```python
from build123d import *

# Parameters (mm, degrees)
F1_DEPTH  = 50.8
F2_R      = 31.75
F3_DEPTH  = 19.05
F4_R      = 12.7
F5_DEPTH  = 38.1
F6_R      = 22.225
F7_DEPTH  = 25.4
F11_R     = 10.16
F12_DEPTH = 25.4


# Not quite as in the source:
# - a fillet or chamfer that OpenCascade refuses, or shapes differently, is made with other operations: its cross-section is extruded or revolved along the edge and cut away or added


with BuildPart() as f1:
    # F0 (on Top) → F1 (new body)
    with BuildSketch(Plane.XY):
        Polygon((76.6512806053, -31.75), (76.6512806053, 31.75), (31.75, 76.6512806053), (-31.75, 76.6512806053), (-76.6512806053, 31.75), (-76.6512806053, -31.75), (-31.75, -76.6512806053), (31.75, -76.6512806053), align=None)
    extrude(amount=F1_DEPTH)

    # F2 (on face) → F3 (cut)
    with BuildSketch(Plane.XY.offset(50.8)):
        Circle(F2_R)
    extrude(amount=-F3_DEPTH, mode=Mode.SUBTRACT)

    # F4 (on face) → F5 (cut)
    with BuildSketch(Plane.XY.offset(50.8)):
        Circle(F4_R)
    extrude(amount=-F5_DEPTH, mode=Mode.SUBTRACT)

    # F6 (on face) → F7 (cut)
    with BuildSketch(Plane.XY.offset(50.8)):
        Circle(F6_R)
    extrude(amount=-F7_DEPTH, mode=Mode.SUBTRACT)

    # F8: fillet of radius 10.16 on 1 edges, made by hand

    # F8_s1 → F8_t2 (revolve)
    with BuildSketch(Plane.XZ):
        with BuildLine():
            ThreePointArc((31.75, 41.8901368334), (28.9953089065, 34.9340603531), (22.225, 31.75))
            Line((22.225, 31.75), (31.75, 31.75))
            Line((31.75, 31.75), (31.75, 41.8901368334))
        make_face()
    revolve(axis=Axis((0, 0, 31.75), (0, 0, 1)))

    # F9: fillet of radius 10.16 on 1 edges, made by hand

    # F9_s1 → F9_t2 (revolve)
    with BuildSketch(Plane.XZ):
        with BuildLine():
            ThreePointArc((22.225, 31.75), (18.4860405842, 27.1357730325), (12.8064279214, 25.4))
            Line((12.8064279214, 25.4), (22.225, 25.4))
            Line((22.225, 25.4), (22.225, 31.75))
        make_face()
    revolve(axis=Axis((0, 0, 25.4), (0, 0, 1)))

    # F10: chamfer of 10.16 on 1 edges, made by hand

    # F10_s1 → F10_t2 (revolve, cut)
    with BuildSketch(Plane.XZ):
        with BuildLine():
            Line((26.0358422648, 32.838882269), (19.9865565056, 28.4792884435))
            Line((19.9865565056, 28.4792884435), (19.8363599068, 28.6161504971))
            ThreePointArc((19.8363599068, 28.6161504971), (21.1312925718, 30.0979038097), (22.0366285584, 31.8262))
            Line((22.0366285584, 31.8262), (22.2123, 31.9528027367))
            ThreePointArc((22.2123, 31.9528027367), (24.1382310347, 32.2649415193), (25.9535194466, 33.0246595378))
            Line((25.9535194466, 33.0246595378), (26.0358422648, 32.838882269))
        make_face()
    revolve(axis=Axis((0, 0, 31.75), (0, 0, 1)), mode=Mode.SUBTRACT)

    # F11 (on face) → F12 (join)
    with BuildSketch(Plane.XY.offset(12.7)):
        Circle(F11_R)
    extrude(amount=F12_DEPTH)


solid = f1.part
```
Can you work these out from the model? Positions are in its coordinate system, mm. A direction names the side the tool comes from. Give positions to 0.01 mm unless a question says otherwise; leave off trailing zeros. Write each loop counter-clockwise with the first axis right and the second up, starting at its lowest first coordinate (ties: lowest second). Pieces come first, ordered by that corner, then holes. Notation, with made-up numbers: (12, -29.5) - (54, -29.5) arc R20 ccw to (54, 2.5) - close; hole circle Ø5 at (68.25, -22). An arc over 180 degrees is marked (long way). Write item = value, one per line. Start each with the question number.
1. On a 3-axis mill with a long thin cutter (end or side, diameter ignored), from which of +Z, -Z, +X, -X, +Y, -Y can I reach the whole of each face in a straight line? I mean faces 4 (the face through (-6.883, -30.995, 46.407)), 5 (the face through (33, 1, 50.8)). Say none if no direction works.
2. Imagine slicing it at B-B (y = 0). Please give me the cut outline in (x, z), and give its area (3 significant figures).
3. For pin 1 (10 mm diameter, centred on y = -33.5, z = 13, fed in from -X); pin 2 (1 mm diameter, centred on y = -60, z = 14, fed in from -X); pin 3 (6 mm diameter, centred on x = -0.5, y = -1, fed in from +Z); pin 4 (10 mm diameter, centred on x = 58.5, z = 26, fed in from -Y), each with a flat end and sliding along its axis, tell me the tip position at first contact or that it passes through.
4. Imagine slicing it at A-A (z = 35.5). Please give me the cut outline in (x, y).
5. Imagine slicing it at D-D (y = 47). Please give me the cut outline in (x, z), and give its area (3 significant figures).
6. Thinking about a two-plate mould opening in Y: for faces 1 (the face through (76.651, 0, 25)), 2 (the face through (-54.5, -53.9, 25)), 3 (the face through (0, 0, 38.1)), which applies, released by +Y, released by -Y, zero draft, split by the parting line, or undercut?
7. Please list where these lines run through material, in increasing order: line 1 (Y direction, x = 0, z = 16); line 2 (Y direction, x = 4.5, z = 16); line 3 (Y direction, x = 0, z = 48.5).
Worked answers:
q1.face_4 = +Z
q1.face_5 = +Z, +X, -X, +Y, -Y
q2.outline = (-76.65, 0) - (76.65, 0) - (76.65, 50.8) - (31.75, 50.8) - (31.75, 41.89) arc R10.16 cw to (25.71, 32.6) - (20.32, 28.72) arc R10.16 cw to (12.81, 25.4) - (12.7, 25.4) - (12.7, 12.7) - (10.16, 12.7) - (10.16, 38.1) - (-10.16, 38.1) - (-10.16, 12.7) - (-12.7, 12.7) - (-12.7, 25.4) - (-12.81, 25.4) arc R10.16 cw to (-20.32, 28.72) - (-25.71, 32.6) arc R10.16 cw to (-31.75, 41.89) - (-31.75, 50.8) - (-76.65, 50.8) - close
q2.area = 6,560 mm2
q3.pin_1 = -76.65
q3.pin_2 = -48.9
q3.pin_3 = 38.1
q3.pin_4 = -54.9
q4.outline = (-76.65, -31.75) - (-31.75, -76.65) - (31.75, -76.65) - (76.65, -31.75) - (76.65, 31.75) - (31.75, 76.65) - (-31.75, 76.65) - (-76.65, 31.75) - close; circle Ø20.32 at (0, 0); hole circle Ø58.98 at (0, 0)
q5.outline = (-61.4, 0) - (61.4, 0) - (61.4, 50.8) - (-61.4, 50.8) - close
q5.area = 6,240 mm2
q6.face_1 = zero draft
q6.face_2 = released by -Y
q6.face_3 = undercut
q7.line_1 = -76.65 to -12.7, -10.16 to 10.16, 12.7 to 76.65
q7.line_2 = -76.65 to -11.88, -9.11 to 9.11, 11.88 to 76.65
q7.line_3 = -76.65 to -31.75, 31.75 to 76.65
